Geometry check sheet. Reference: the model listing, model coordinates, mm. A direction names the side the tool comes from. Round coordinates to 2 decimals unless told otherwise and drop trailing zeros. Order: outer loops, then holes, each group sorted by start corner. A loop starts at its lowest first (then second) coordinate and runs counter-clockwise, first axis right, second up. Notation, with made-up numbers: (2.5, 37.25) -> (46.5, 37.25) arc R17 ccw to (46.5, 49.25) -> close; hole circle Ø5 at (-23, 31). An arc over 180 degrees is marked (long way). Use a Markdown table: item, result. Add a question column.
Item 1: Sectioned sample at B-B, the plane z = 0.75. Record the cut outline in (x, y), and give its area (3 significant figures).
Item 2: Sectioned sample at A-A, the plane x = -3.25. Record the cut outline in (y, z).
Item 3: Sectioned sample at D-D, the plane y = 11. Record the cut outline in (x, z), and give its area (3 significant figures).
Item 4: Mould release check, pull along X, two halves, no side actions. Record for faces 4 (the flat face through (-8, 2.8, 2)), 5 (the flat face through (0, 14, 2)), 6 (the flat face through (-13.024, 4.033, 2.465)), 7 (the flat face through (-2, 8, 5)): pulls with the +X half, pulls with the -X half, needs draft (parallel to the pull), parting line crosses it, or undercut.
Item 5: Material ranges on probe 1 along X at (y, z) = (14.5, 2.7); probe 2 along Y at (x, z) = (-8.25, 4.65); probe 3 along Y at (x, z) = (-6.25, 3.2), recorded low to high. Write a range as [from, to].
Item 6: Sectioned sample at C-C, the plane x = -9. Record the cut outline in (y, z).
Item 7: Gauge pin test, flat ends, axial feed: pin 1 Ø2.5 at (x, z) = (-13, 3) entering from +Y; pin 2 Ø1.9 at (y, z) = (-1, 2.5) entering from +X; pin 3 Ø2.5 at (y, z) = (9, 3) entering from -X. Record the tip position at first contact, or that the pin passes through.
Item 8: Set-up check for faces 1 (the flat face through (-5, 26.8, 2)), 2 (the flat face through (-7, 0, 2)), 3 (the flat face through (-17.461, 0, 2)): record each of +Z, -Z, +X, -X, +Y, -Y from which the full face is reachable in a straight line by a thin tool's end or side.
from build123d import *

# Parameters (mm, degrees)
F1_DEPTH    = 5
F2_T1_DEPTH = 29.4948974279
F2_T3_DEPTH = 30


# Not quite as in the source:
# - a fillet or chamfer that OpenCascade refuses, or shapes differently, is made with other operations: its cross-section is extruded or revolved along the edge and cut away or added


with BuildPart() as f1:
    # F0 (on Top) → F1 (new body)
    with BuildSketch(Plane.XY):
        with BuildLine():
            Line((-17.4608190332, -5.4), (-10.4608190332, -5.4))
            Line((-10.4608190332, -5.4), (-11.7008190332, -2.4))
            Line((-11.7008190332, -2.4), (-14.1008190332, -2.4))
            Line((-14.1008190332, -2.4), (-14.1008190332, 0))
            Line((-14.1008190332, 0), (0, 0))
            Line((0, 0), (0, 28.3))
            Line((0, 28.3), (-2.7189972619, 28.3))
            ThreePointArc((-2.7189972619, 28.3), (-4.184287104, 28.1646631001), (-5.6, 27.7632314196))
            Line((-5.6, 27.7632314196), (-6.8, 27.3))
            Line((-6.8, 27.3), (-6.8, 26.8))
            Line((-6.8, 26.8), (-2.8, 26.8))
            Line((-2.8, 26.8), (-2.8, 2.8))
            Line((-2.8, 2.8), (-12.6, 2.8))
            Line((-12.6, 2.8), (-13.4608190332, 5.3))
            Line((-13.4608190332, 5.3), (-17.4608190332, 5.3))
            Line((-17.4608190332, 5.3), (-17.4608190332, -5.4))
        make_face()
    extrude(amount=F1_DEPTH)

    # F2: fillet of radius 5 on 2 edges, made by hand

    # F2_s2 → F2_t1 (cut)
    with BuildSketch(Plane.XY.offset(-12.2474487139)):
        with BuildLine():
            ThreePointArc((-13.4608190332, 5.3), (-16.3338023794, 3.5632981746), (-17.4608190332, 0.4010205144))
            Line((-17.4608190332, 0.4010205144), (-17.4608190332, 5.3))
            Line((-17.4608190332, 5.3), (-13.4608190332, 5.3))
        make_face()
    extrude(amount=F2_T1_DEPTH, mode=Mode.SUBTRACT)

    # F2_s4 → F2_t3 (cut)
    with BuildSketch(Plane.XY.offset(-12.5)):
        with BuildLine():
            ThreePointArc((-17.4608190332, -0.4), (-15.9963529392, -3.9355339059), (-12.4608190332, -5.4))
            Line((-12.4608190332, -5.4), (-17.4608190332, -5.4))
            Line((-17.4608190332, -5.4), (-17.4608190332, -0.4))
        make_face()
    extrude(amount=F2_T3_DEPTH, mode=Mode.SUBTRACT)


solid = f1.part
Found:
| question | item | result |
|---|---|---|
| 1 | outline | (-17.46, -0.4) arc R5 ccw to (-12.46, -5.4) -> (-10.46, -5.4) -> (-11.7, -2.4) -> (-14.1, -2.4) -> (-14.1, 0) -> (0, 0) -> (0, 28.3) -> (-2.72, 28.3) arc R8 ccw to (-5.6, 27.76) -> (-6.8, 27.3) -> (-6.8, 26.8) -> (-2.8, 26.8) -> (-2.8, 2.8) -> (-12.6, 2.8) -> (-13.46, 5.3) arc R5 ccw to (-17.46, 0.4) -> close |
| 1 | area | 153 mm2 |
| 2 | outline | (0, 0) -> (2.8, 0) -> (2.8, 5) -> (0, 5) -> close; (26.8, 0) -> (28.28, 0) -> (28.28, 5) -> (26.8, 5) -> close |
| 3 | outline | (-2.8, 0) -> (0, 0) -> (0, 5) -> (-2.8, 5) -> close |
| 3 | area | 14.0 mm2 |
| 4 | face 4 | undercut |
| 4 | face 5 | pulls with the +X half |
| 4 | face 6 | undercut |
| 4 | face 7 | needs draft |
| 5 | probe 1 | x = [-2.8, 0] |
| 5 | probe 2 | y = [0, 2.8] |
| 5 | probe 3 | y = [0, 2.8], [26.8, 27.51] |
| 6 | outline | (0, 0) -> (2.8, 0) -> (2.8, 5) -> (0, 5) -> close |
| 7 | pin 1 | stops at y = 5.3 |
| 7 | pin 2 | stops at x = -14.1 |
| 7 | pin 3 | stops at x = -2.8 |
| 8 | face 1 | +Z, -Z, -X |
| 8 | face 2 | +Z, -Z, +X |
| 8 | face 3 | +Z, -Z, -X, +Y, -Y |
